from build123d import *

# Parameters (mm, degrees)
EXTRUDE_1_DEPTH     = 100
CUT_EXTRUDE_1_REACH = 5
SKETCH_2_R          = 5


with BuildPart() as part:
    # Эскиз1 → Бобышка-Вытянуть1 (new body)
    with BuildSketch(Plane.XY):
        Polygon((0, 0), (0, 40), (3, 40), (3, 3), (40, 3), (40, 0), align=None)
    extrude(amount=EXTRUDE_1_DEPTH)

    # Эскиз2 → Вырез-Вытянуть1 (cut, up to next)
    with BuildSketch(Plane(origin=(0, 3, 0), x_dir=(1, 0, 0), z_dir=(0, 1, 0)), mode=Mode.PRIVATE) as cut_extrude_1_sk1:
        with Locations((21.5, -20)):
            Circle(SKETCH_2_R)
    cut_extrude_1_tool1 = extrude(cut_extrude_1_sk1.sketch, amount=-CUT_EXTRUDE_1_REACH, mode=Mode.PRIVATE) & part.part
    add(cut_extrude_1_tool1.solids().sort_by_distance((21.5, 3, 20))[0], mode=Mode.SUBTRACT)
    # Эскиз2 → Вырез-Вытянуть1 (cut, up to next)
    with BuildSketch(Plane(origin=(0, 3, 0), x_dir=(1, 0, 0), z_dir=(0, 1, 0)), mode=Mode.PRIVATE) as cut_extrude_1_sk2:
        with Locations((21.5, -80)):
            Circle(SKETCH_2_R)
    cut_extrude_1_tool2 = extrude(cut_extrude_1_sk2.sketch, amount=-CUT_EXTRUDE_1_REACH, mode=Mode.PRIVATE) & part.part
    add(cut_extrude_1_tool2.solids().sort_by_distance((21.5, 3, 80))[0], mode=Mode.SUBTRACT)


solid = part.part
For this review, take the finished solid that the model builds, in its own axes (mm). A direction names the side the tool comes from. Give positions to 0.01 mm unless a question says otherwise; leave off trailing zeros. Loops run counter-clockwise (first coordinate to the right, second up) from the corner with the lowest first, then second, coordinate; pieces in that order, holes last. Notation, with made-up numbers: (-8, 79) - (15, 79) arc R18 ccw to (15, 103) - close; hole circle Ø7 at (-37.75, 70). An arc over 180 degrees is marked (long way). Write each question's results on one line, items separated by ' | '.
(1) For line 1 along Z through (x, y) = (21.5, 2.35); line 2 along X through (y, z) = (1.6, 20); line 3 along X through (y, z) = (23, 47), list the stretches that pass through material, from the lowest coordinate up.
Conclusion:
line 1: 0 to 15, 25 to 75, 85 to 100 | line 2: 0 to 16.5, 26.5 to 40 | line 3: 0 to 3
(2) For pin 1 Ø8 at (x, z) = (21.5, 20) entering from +Y, flat-tipped, find the tip position at first contact; note if it passes through.
Conclusion:
pin 1: through
(3) Take a section at A-A (x = 21.5). Give the boundary of the cut face in (y, z).
Conclusion:
outline: (0, 0) - (3, 0) - (3, 15) - (0, 15) - close; (0, 25) - (3, 25) - (3, 75) - (0, 75) - close; (0, 85) - (3, 85) - (3, 100) - (0, 100) - close
(4) Take a section at C-C (z = 59.5). Give the boundary of the cut face in (x, y), then the cut area to 3 significant figures.
Conclusion:
outline: (0, 0) - (40, 0) - (40, 3) - (3, 3) - (3, 40) - (0, 40) - close | area: 231 mm^2
(5) Take a section at D-D (y = 14). Give the boundary of the cut face in (x, z), then the cut area to 3 significant figures.
Conclusion:
outline: (0, 0) - (3, 0) - (3, 100) - (0, 100) - close | area: 300 mm^2
(6) Take a section at B-B (z = 80). Give the boundary of the cut face in (x, y), then the cut area to 3 significant figures.
Conclusion:
outline: (0, 0) - (16.5, 0) - (16.5, 3) - (3, 3) - (3, 40) - (0, 40) - close; (26.5, 0) - (40, 0) - (40, 3) - (26.5, 3) - close | area: 201 mm^2
(7) Draft analysis for pull direction X (two halves, no side actions). For faces 3 (the flat face through (3, 22, 49)), 4 (the flat face through (11, 2, 0)), 5 (the cylindrical face through (20.42, 1.52, 84.88)), 6 (the cylindrical face through (20.42, 1.52, 24.88)), state which applies: +X half, -X half, draft (parallel to the pull), parting line (faces both ways), or undercut.
Conclusion:
face 3: +X half | face 4: draft | face 5: undercut | face 6: undercut
(8) For faces 1 (the flat face through (0, 20, 49)), 2 (the flat face through (21, 3, 49)), list the 3-axis set-ups (+Z, -Z, +X, -X, +Y, -Y) from which the entire face can be reached by the end or side of a thin tool; tool diameter is ignored.
Conclusion:
face 1: +Z, -Z, -X, +Y, -Y | face 2: +Z, -Z, +X, +Y
